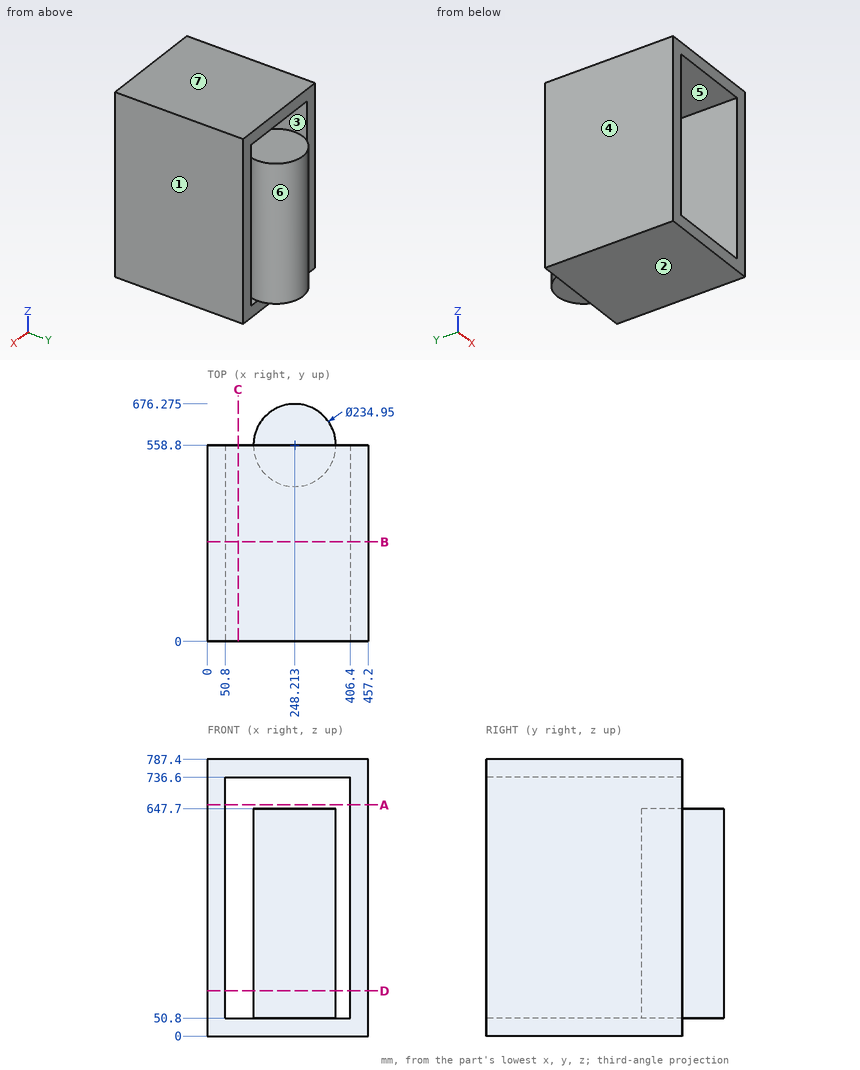
Study the drawing (mm; zero at the part's minimum x, y, z) and answer. A direction names the side the tool comes from. Give positions to 0.01 mm unless a question says otherwise; leave off trailing zeros. Write each loop counter-clockwise with the first axis right and the second up, starting at its lowest first coordinate (ties: lowest second). Pieces come first, ordered by that corner, then holes. Notation, with made-up numbers: (-7, 73) - (3, 73) arc R16 ccw to (3, 102) - close; hole circle Ø1 at (65.25, 37.25). An arc over 180 degrees is marked (long way). Use CSV: the item, a comma, the result in double quotes. Start each with the question number.
(1) For the marked faces 5, 6 and 7, determine the directions among +Z, -Z, +X, -X, +Y, -Y from which every point of the face is accessible in a straight line to the end or side of a thin tool.
(2) Find section C-C (x = 87). Give the vertices of the cut face in (y, z), plus the area to 3 significant figures.
(3) Find section D-D (z = 128.5). Count the separate pieces of the cut face and the enclosed holes in it, plus the area to 3 significant figures.
(4) Find section A-A (z = 658.5). Give the vertices of the cut face in (x, y), plus the area to 3 significant figures.
(5) Find section B-B (y = 284). Give the vertices of the cut face in (x, z), plus the area to 3 significant figures.
(6) Consider line 1 along X through (y, z) = (225, 87); line 2 along Z through (x, y) = (97.5, 74); line 3 along X through (y, z) = (501.5, 609) (1 decimal). Determine where each line is inside the solid, lowest interval first.
(7) Given P1, Ø12, axis at x = 309.5, z = 173, coming from the -Y side; P2, Ø12, axis at x = 204.5, z = 451, coming from the -Y side; P3, Ø2, axis at x = 184.5, z = 130.5, coming from the +Y side (1 decimal); P4, Ø5, axis at x = 286.5, y = 292, coming from the -Z side, each flat-ended and moving along its own axis, determine where each tip first touches the part or whether it passes through.
(8) Determine the mould class of the marked faces 1, 2, 3 and 4 for opening direction X: +X half, -X half, draft (parallel to the pull), parting line (faces both ways), or undercut.
Findings below:
1,face 5,"+Y, -Y"
1,face 6,"none"
1,face 7,"+Z, +X, -X, +Y, -Y"
2,outline,"(0, 0) - (558.8, 0) - (558.8, 50.8) - (0, 50.8) - close; (0, 736.6) - (558.8, 736.6) - (558.8, 787.4) - (0, 787.4) - close"
2,area,"56,800 mm2"
3,separate pieces,"3"
3,enclosed holes,"0"
3,area,"100,000 mm2"
4,outline,"(0, 0) - (50.8, 0) - (50.8, 558.8) - (0, 558.8) - close; (406.4, 0) - (457.2, 0) - (457.2, 558.8) - (406.4, 558.8) - close"
4,area,"56,800 mm2"
5,outline,"(0, 0) - (457.2, 0) - (457.2, 787.4) - (0, 787.4) - close; hole (50.8, 50.8) - (406.4, 50.8) - (406.4, 736.6) - (50.8, 736.6) - close"
5,area,"116,000 mm2"
6,line 1,"0 to 50.8, 406.4 to 457.2"
6,line 2,"0 to 50.8, 736.6 to 787.4"
6,line 3,"0 to 50.8, 145.7 to 350.8, 406.4 to 457.2"
7,P1,"y = 455.15"
7,P2,"y = 447.54"
7,P3,"y = 658.1"
7,P4,"z = 0"
8,face 1,"+X half"
8,face 2,"draft"
8,face 3,"undercut"
8,face 4,"-X half"
